from build123d import *

# Parameters (mm, degrees)
F1_DEPTH       = 10
F2_W           = 45
F2_H           = 10
F3_DEPTH       = 10
F4_R           = 0.5
F5_DEPTH       = 10
F6_R           = 2.1
F7_DEPTH       = 2.5
F8_T1_DEPTH    = 10
F8_T3_DEPTH    = 43.0998702926
F9_T1_DEPTH    = 10
F9_T3_DEPTH    = 15.8191503542
F9_T5_DEPTH    = 16.25
F9_T7_DEPTH    = 36.3051320704
F11_DEPTH      = 5
F11_TAPER      = -30
F11_DEPTH_BACK = 5


# Not quite as in the source:
# - a fillet or chamfer that OpenCascade refuses, or shapes differently, is made with other operations: its cross-section is extruded or revolved along the edge and cut away or added


with BuildPart() as f1:
    # F0 (on Top) → F1 (new body)
    with BuildSketch(Plane.XY):
        with BuildLine():
            ThreePointArc((0, -1.25), (0.8838834765, -0.8838834765), (1.25, 0))
            ThreePointArc((1.25, 0), (0.8838834765, 0.8838834765), (0, 1.25))
            ThreePointArc((0, 1.25), (-1.25, 0), (0, -1.25))
        make_face()
        with BuildLine():
            ThreePointArc((0, -1.25), (-1.25, 0), (0, 1.25))
            ThreePointArc((0, 1.25), (-3.9258033341, 0.8039751431), (-7.6514917116, -0.5113636364))
            ThreePointArc((-7.6514917116, -0.5113636364), (-3.8435305739, -1.0649126927), (0, -1.25))
        make_face()
        with BuildLine():
            ThreePointArc((-7.6514917116, -0.5113636364), (-3.9258033341, 0.8039751431), (0, 1.25))
            ThreePointArc((0, 1.25), (-37.5, 38.75), (0, 76.25))
            Line((0, 76.25), (0, 78.75))
            ThreePointArc((0, 78.75), (-39.8149126927, 42.5935305739), (-7.6514917116, -0.5113636364))
        make_face()
        with BuildLine():
            ThreePointArc((-0.5, -31.2416643506), (-14.9979159429, -15.9999652609), (0, -1.25))
            ThreePointArc((0, -1.25), (-3.8435305739, -1.0649126927), (-7.6514917116, -0.5113636364))
            ThreePointArc((-7.6514917116, -0.5113636364), (-17.3284932243, -18.69403817), (-3, -33.4909396496))
            Line((-3, -33.4909396496), (-3, -31.2416643506))
            Line((-3, -31.2416643506), (-0.5, -31.2416643506))
        make_face()
        with BuildLine():
            Line((-0.5, -33.7428556845), (-0.5, -31.2416643506))
            Line((-0.5, -31.2416643506), (-3, -31.2416643506))
            Line((-3, -31.2416643506), (-3, -33.4909396496))
            ThreePointArc((-3, -33.4909396496), (-1.7545271221, -33.661824562), (-0.5, -33.7428556845))
        make_face()
        with BuildLine():
            ThreePointArc((-0.5, -33.7428556845), (-1.7545271221, -33.661824562), (-3, -33.4909396496))
            Line((-3, -33.4909396496), (-3, -43.7428556845))
            Line((-3, -43.7428556845), (-0.5, -43.7428556845))
            Line((-0.5, -43.7428556845), (-0.5, -33.7428556845))
        make_face()
    extrude(amount=F1_DEPTH)

    # F2 (on Top) → F3 (cut, through all)
    with BuildSketch(Plane.XY):
        with Locations((0, 73.75)):
            Rectangle(F2_W, F2_H)
    extrude(amount=F3_DEPTH, mode=Mode.SUBTRACT)

    # F4 (on face) → F5 (cut, through all)
    with BuildSketch(Plane.XY.offset(10)):
        Circle(F4_R)
    extrude(amount=-F5_DEPTH, mode=Mode.SUBTRACT)

    # F6 (on face) → F7 (cut, through all)
    with BuildSketch(Plane(origin=(-3, 0, 0), x_dir=(0, -1, 0), z_dir=(-1, 0, 0))):
        with Locations((38.6168976671, 5)):
            Circle(F6_R)
    extrude(amount=-F7_DEPTH, mode=Mode.SUBTRACT)

    # F8: fillet of radius 5 on 2 edges, made by hand

    # F8_s2 → F8_t1 (join)
    with BuildSketch(Plane.XY):
        with BuildLine():
            ThreePointArc((-13.8860405137, -5.5997474747), (-13.0142523991, -1.2990941124), (-15.8697605871, 2.0328282828))
            ThreePointArc((-15.8697605871, 2.0328282828), (-11.8292246388, 0.5391449396), (-7.6514917116, -0.5113636364))
            ThreePointArc((-7.6514917116, -0.5113636364), (-11.0652264374, -2.6923171637), (-13.8860405137, -5.5997474747))
        make_face()
    extrude(amount=F8_T1_DEPTH)

    # F8_s4 → F8_t3 (cut)
    with BuildSketch(Plane.XY.offset(-16.5499351463)):
        with BuildLine():
            ThreePointArc((-22.5, 68.75), (-25.2284691248, 68.9356152516), (-27.6464669917, 67.6580068991))
            ThreePointArc((-27.6464669917, 67.6580068991), (-25.1595214868, 69.8465991477), (-22.5, 71.8218913883))
            Line((-22.5, 71.8218913883), (-22.5, 68.75))
        make_face()
    extrude(amount=F8_T3_DEPTH, mode=Mode.SUBTRACT)

    # F9: fillet of radius 1.25 on 5 edges, made by hand

    # F9_s2 → F9_t1 (join)
    with BuildSketch(Plane.XY):
        with BuildLine():
            ThreePointArc((-3, -34.5119823677), (-3.2710549896, -33.73470078), (-3.9666666667, -33.2945168766))
            ThreePointArc((-3.9666666667, -33.2945168766), (-3.4847175764, -33.3995406181), (-3, -33.4909396496))
            Line((-3, -33.4909396496), (-3, -34.5119823677))
        make_face()
    extrude(amount=F9_T1_DEPTH)

    # F9_s4 → F9_t3 (cut)
    with BuildSketch(Plane.XY.offset(-2.9095751771)):
        with BuildLine():
            ThreePointArc((-1.6153846154, -31.1627640813), (-0.8197394906, -31.5705600619), (-0.5, -32.4054944214))
            Line((-0.5, -32.4054944214), (-0.5, -31.2416643506))
            ThreePointArc((-0.5, -31.2416643506), (-1.0584277637, -31.2126110913), (-1.6153846154, -31.1627640813))
        make_face()
    extrude(amount=F9_T3_DEPTH, mode=Mode.SUBTRACT)

    # F9_s6 → F9_t5 (cut)
    with BuildSketch(Plane.XY.offset(-3.125)):
        with BuildLine():
            ThreePointArc((-0.5, -42.4928556845), (-0.8661165235, -43.376739161), (-1.75, -43.7428556845))
            Line((-1.75, -43.7428556845), (-0.5, -43.7428556845))
            Line((-0.5, -43.7428556845), (-0.5, -42.4928556845))
        make_face()
        with BuildLine():
            ThreePointArc((-1.75, -43.7428556845), (-2.6338834765, -43.376739161), (-3, -42.4928556845))
            Line((-3, -42.4928556845), (-3, -43.7428556845))
            Line((-3, -43.7428556845), (-1.75, -43.7428556845))
        make_face()
    extrude(amount=F9_T5_DEPTH, mode=Mode.SUBTRACT)

    # F9_s8 → F9_t7 (cut)
    with BuildSketch(Plane.XY.offset(-13.1525660352)):
        with BuildLine():
            ThreePointArc((-25.9185526928, 65.8512661385), (-25.8791274069, 67.6185918599), (-27.6464530598, 67.658020223))
            ThreePointArc((-27.6464530598, 67.658020223), (-25.2284596959, 68.9356172522), (-22.5, 68.75))
            ThreePointArc((-22.5, 68.75), (-24.2526230688, 67.3517529932), (-25.9185526928, 65.8512661385))
        make_face()
    extrude(amount=F9_T7_DEPTH, mode=Mode.SUBTRACT)

    # F10 (on Front) → F11 (cut, two sides)
    with BuildSketch(Plane.XZ) as f11_sk:
        Polygon((1.5, 0.0747326796), (1.5, 4.9252673204), (-1.6606699079, 2.5), align=None)
        Polygon((1.5, 9.9252673204), (-1.6606699079, 7.5), (1.5, 5.0747326796), align=None)
    extrude(amount=-F11_DEPTH, taper=F11_TAPER, mode=Mode.SUBTRACT)
    extrude(f11_sk.sketch, amount=F11_DEPTH_BACK, mode=Mode.SUBTRACT)


solid = f1.part
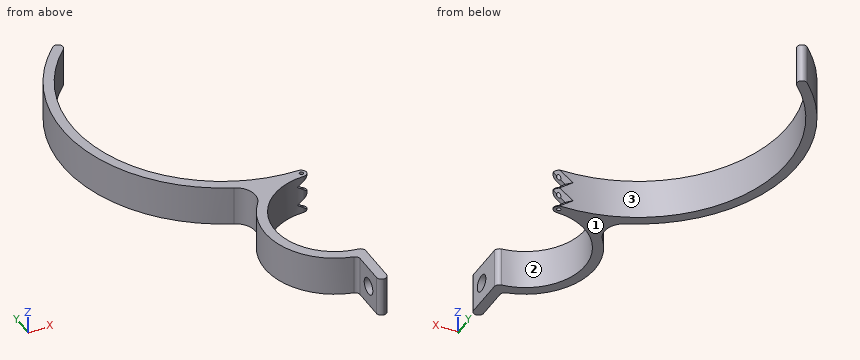
For this review, take the finished solid that the model builds, in its own axes (mm). Face numbers are marked on the shaded views. Round coordinates to 2 decimals unless told otherwise and drop trailing zeros. Loops run counter-clockwise (first coordinate to the right, second up) from the corner with the lowest first, then second, coordinate; pieces in that order, holes last. Notation, with made-up numbers: (-36, -30) - (15, -30) arc R21 cw to (15, 5) - close; hole circle Ø5 at (16, 46.25). An arc over 180 degrees is marked (long way). Put each result on its own line as item: value. Start each with the question number.
1. Mouldability with a two-part tool opening along Y and no side actions: class the marked faces 1, 2 and 3 as +Y half, -Y half, draft (parallel to the pull), parting line (faces both ways), or undercut.
2. For probe 1 along X at (y, z) = (-37, 7.75); probe 2 along X at (y, z) = (0, 0.5); probe 3 along Y at (x, z) = (-4, 6.75), list the stretches that pass through material, from the lowest coordinate up. Write a range as [from, to].
3. Insertion check: P1, Ø2, axis at y = 30, z = 3.5, coming from the -X side; P2, Ø3, axis at y = 43.5, z = 5, coming from the -X side; P3, Ø5, axis at x = -9, z = 6.5, coming from the -Y side. Each pin has a flat end and moves straight along its axis. Give the tip position at first contact, or say it passes through.
4. Consider section A-A on y = -16.25. State the section outline as (x, z) points, plus the area to 3 significant figures.
5. Consider section B-B on x = -22.5. State the section outline as (y, z) points.
Result sheet:
1. face 1: draft
1. face 2: undercut
1. face 3: undercut
2. probe 1: [-3, -0.5]
2. probe 2: [-13.56, -0.5], [0.5, 0.95]
2. probe 3: [-33.29, -30.71], [-1.79, 1.46]
3. P1: x = -39.24
3. P2: x = -39.87
3. P3: y = -32.5
4. outline: (-17.5, 0) - (-15, 0) - (-15, 10) - (-17.5, 10) - close
4. area: 25.0 mm^2
5. outline: (5.68, 0) - (8.75, 0) - (8.75, 10) - (5.68, 10) - close
